```python
from build123d import *

# Parameters (mm, degrees)
F0_W      = 126.176424
F0_H      = 112.621017
F1_DEPTH  = 25.4
F2_W      = 26.31655
F2_H      = 15.193862
F3_DEPTH  = 25.4
F4_W      = 34.140256
F4_H      = 21.598417
F5_DEPTH  = 25.4
F7_W      = 34.864582
F7_H      = 18.686838
F8_DEPTH  = 25.4
F6_W      = 39.589775
F6_H      = 19.492015
F11_DEPTH = 25.4
F9_W      = 17.070128
F9_H      = 21.598417
F12_DEPTH = 50.8
F10_W     = 13.158275
F10_H     = 15.193862
F13_DEPTH = 50.8
F14_W     = 17.432291
F14_H     = 18.686838
F15_DEPTH = 50.8
F16_W     = 19.794888
F16_H     = 19.492015
F17_DEPTH = 50.8


with BuildPart() as f1:
    # F0 (on Top) → F1 (new body)
    with BuildSketch(Plane.XY):
        with Locations((-4.600737, 5.364046)):
            Rectangle(F0_W, F0_H)
    extrude(amount=F1_DEPTH)

    # F2 (on face) → F3 (join)
    with BuildSketch(Plane(origin=(0, 0, 0), x_dir=(1, 0, 0), z_dir=(0, 0, -1))):
        with Locations((35.497902, 25.018883)):
            Rectangle(F2_W, F2_H)
    extrude(amount=F3_DEPTH)

    # F4 (on face) → F5 (join)
    with BuildSketch(Plane(origin=(0, 0, 0), x_dir=(1, 0, 0), z_dir=(0, 0, -1))):
        with Locations((-41.06454, 35.200375)):
            Rectangle(F4_W, F4_H)
    extrude(amount=F5_DEPTH)

    # F7 (on face) → F8 (join)
    with BuildSketch(Plane(origin=(0, 0, 0), x_dir=(1, 0, 0), z_dir=(0, 0, -1))):
        with Locations((36.498174, -44.728223)):
            Rectangle(F7_W, F7_H)
    extrude(amount=F8_DEPTH)

    # F6 (on face) → F11 (join)
    with BuildSketch(Plane(origin=(0, 0, 0), x_dir=(1, 0, 0), z_dir=(0, 0, -1))):
        with Locations((-32.867522, -44.407618)):
            Rectangle(F6_W, F6_H)
    extrude(amount=F11_DEPTH)

    # F9 (on face) → F12 (join)
    with BuildSketch(Plane(origin=(0, 0, -25.4), x_dir=(1, 0, 0), z_dir=(0, 0, -1))):
        with Locations((-49.599604, 35.200375)):
            Rectangle(F9_W, F9_H)
    extrude(amount=F12_DEPTH)

    # F10 (on face) → F13 (join)
    with BuildSketch(Plane(origin=(0, 0, -25.4), x_dir=(1, 0, 0), z_dir=(0, 0, -1))):
        with Locations((42.077039, 25.018883)):
            Rectangle(F10_W, F10_H)
    extrude(amount=F13_DEPTH)

    # F14 (on face) → F15 (join)
    with BuildSketch(Plane(origin=(0, 0, -25.4), x_dir=(1, 0, 0), z_dir=(0, 0, -1))):
        with Locations((45.21432, -44.728223)):
            Rectangle(F14_W, F14_H)
    extrude(amount=F15_DEPTH)

    # F16 (on face) → F17 (join)
    with BuildSketch(Plane(origin=(0, 0, -25.4), x_dir=(1, 0, 0), z_dir=(0, 0, -1))):
        with Locations((-42.764966, -44.407618)):
            Rectangle(F16_W, F16_H)
    extrude(amount=F17_DEPTH)


solid = f1.part
```
Design review of the part built by this model. Coordinates are the model's own, in mm. A direction names the side the tool comes from. Give positions to 0.01 mm unless a question says otherwise; leave off trailing zeros. Order: outer loops, then holes, each group sorted by start corner. A loop starts at its lowest first (then second) coordinate and runs counter-clockwise, first axis right, second up. Notation, with made-up numbers: M 20.5,76.25 L 27.5,76.25 A16 cw 27.5,101.25 Z; hole C 34.25,13.25 d11. An arc over 180 degrees is marked long. One line per question, with ' | ' between items. Start each with the question number.
Q1. We need section D-D (z = -19). Write out the cut boundary in (x, y), plus the area to 3 significant figures.
Q2. For pin 1 Ø21 at (x, z) = (31, -26) entering from -Y; pin 2 Ø6.5 at (y, z) = (-39.5, -11.5) entering from +X; pin 3 Ø11 at (y, z) = (-37, -39.5) entering from +X, all flat-tipped, find the tip position at first contact; note any pin that passes through.
Q3. We need section C-C (y = 50). Write out the cut boundary in (x, z), plus the area to 3 significant figures.
Q4. For L1, parallel to Y at x = 35, z = -9; L2, parallel to X at y = 41, z = -13.5; L3, parallel to X at y = 49, z = -54, list the stretches that pass through material, from the lowest coordinate up. Write a range as [from, to].
Q5. Machinability: for faces 4 (the face through (22.34, -25, -13)), 5 (the face through (48.656, -25, -13)), 6 (the face through (40, 35.385, -29)), which of the approach directions +Z, -Z, +X, -X, +Y, -Y give a long, thin tool a straight path to every point of the face, cutting with its end or side? Answer none if there is none.
Q6. We need section A-A (z = -63). Write out the cut boundary in (x, y), plus the area to 3 significant figures.
Q7. We need section B-B (x = 32). Write out the cut boundary in (y, z).
Q8. The part is to be moulded in two halves that separate along X. For faces 1 (the face through (-32.868, 45, -50)), 2 (the face through (-67.689, 5, 13)), 3 (the face through (53.93, 45, -13)), say which applies: +X half, -X half, draft (parallel to the pull), parting line (faces both ways), or undercut.
Returned:
1) outline: M -58.13,-46 L -23.99,-46 L -23.99,-24.4 L -58.13,-24.4 Z; M -52.66,34.66 L -13.07,34.66 L -13.07,54.15 L -52.66,54.15 Z; M 19.07,35.38 L 53.93,35.38 L 53.93,54.07 L 19.07,54.07 Z; M 22.34,-32.62 L 48.66,-32.62 L 48.66,-17.42 L 22.34,-17.42 Z | area: 2,560 mm2
2) pin 1: y = -32.62 | pin 2: x = -23.99 | pin 3: x = 48.66
3) outline: M -67.69,0 L -52.66,0 L -52.66,-76.2 L -32.87,-76.2 L -32.87,-25.4 L -13.07,-25.4 L -13.07,0 L 19.07,0 L 19.07,-25.4 L 36.5,-25.4 L 36.5,-76.2 L 53.93,-76.2 L 53.93,0 L 58.49,0 L 58.49,25.4 L -67.69,25.4 Z | area: 6,990 mm2
4) L1: [-32.62, -17.42], [35.38, 54.07] | L2: [-52.66, -13.07], [19.07, 53.93] | L3: [-52.66, -32.87], [36.5, 53.93]
5) face 4: -Z, -Y | face 5: -Z, +X, -Y | face 6: -Z, +X
6) outline: M -58.13,-46 L -41.06,-46 L -41.06,-24.4 L -58.13,-24.4 Z; M -52.66,34.66 L -32.87,34.66 L -32.87,54.15 L -52.66,54.15 Z; M 35.5,-32.62 L 48.66,-32.62 L 48.66,-17.42 L 35.5,-17.42 Z; M 36.5,35.38 L 53.93,35.38 L 53.93,54.07 L 36.5,54.07 Z | area: 1,280 mm2
7) outline: M -50.95,0 L -32.62,0 L -32.62,-25.4 L -17.42,-25.4 L -17.42,0 L 35.38,0 L 35.38,-25.4 L 54.07,-25.4 L 54.07,0 L 61.67,0 L 61.67,25.4 L -50.95,25.4 Z
8) face 1: undercut | face 2: -X half | face 3: +X half
